Design review of the part built by this model. Coordinates are the model's own, in mm. Face numbers are marked on the shaded views. A direction names the side the tool comes from. Coordinates: 2 decimals unless noted, no trailing zeros. Loops run counter-clockwise (first coordinate to the right, second up) from the corner with the lowest first, then second, coordinate; pieces in that order, holes last. Notation, with made-up numbers: (6, 26) -> (35, 26) arc R23 ccw to (35, 53) -> close; hole circle Ø2 at (28, 63.25). An arc over 180 degrees is marked (long way). Answer in a Markdown table with one row per item.
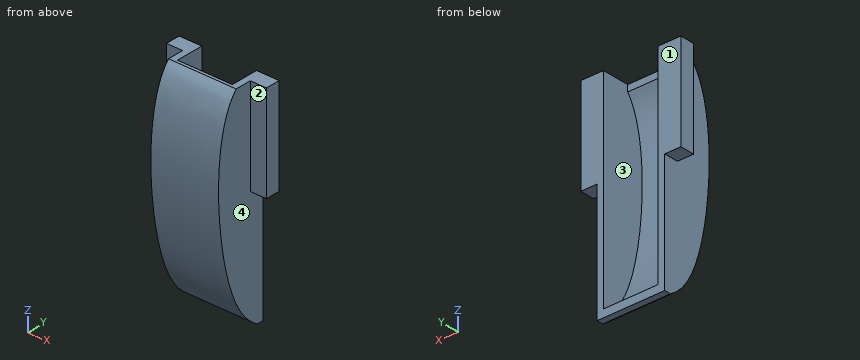
```python
from build123d import *

# Parameters (mm, degrees)
BASEPIEDEAPPOGGIO_START = -10.5
BASEPIEDEAPPOGGIO_DEPTH = 21
LATOSINISTRO_DEPTH      = 2
SCHIZZO3_W              = 5
SCHIZZO3_H              = 4.5
ALETTEAGGANCIO_DEPTH    = 30


# Read off the part's stored shape, not the designer's step: BasePiedeAppoggio
with BuildPart() as part:
    # BasePiedeAppoggio outline → BasePiedeAppoggio (new body)
    with BuildSketch(Plane(origin=(0, 0, 0), x_dir=(0, 0, -1), z_dir=(1, 0, 0)).offset(BASEPIEDEAPPOGGIO_START)):
        with BuildLine():
            Line((-67, -6.58541733), (-67, -7.5))
            add(Edge.make_bspline(
                [(-67, -7.5), (-60, -14), (-44, -17), (-14, -13), (-5, -8), (0, 0)],
                knots=[0, 0, 0, 0, 0, 0, 1, 1, 1, 1, 1, 1], degree=5))
            Line((0, 0), (0, 2))
            Line((0, 2), (-2.409917527, 2))
            Line((-2.409917527, 2), (-2.409917527, 0))
            add(Edge.make_bspline(
                [(-2.409917527, 0), (-2.667324323, -0.353402954), (-3.476108464, -1.377540434), (-5.718312008, -3.574118885), (-10.497685703, -6.435761001), (-19.037438877, -9.233820798), (-29.572047533, -11.136431528), (-38.966676556, -11.799385995), (-46.135832891, -11.693755764), (-51.166703498, -11.28631183), (-55.693282116, -10.549034431), (-58.932001396, -9.671882802), (-61.157085706, -8.829738395), (-62.633910182, -8.137838289), (-63.931461685, -7.382278902), (-64.645771008, -6.869387628), (-65, -6.58541733)],
                knots=[0.030225408, 0.030225408, 0.030225408, 0.030225408, 0.061229523, 0.122459046, 0.244918093, 0.367377139, 0.489836186, 0.612295232, 0.673524756, 0.734754279, 0.795983802, 0.857213325, 0.887828087, 0.918442849, 0.94905761, 0.979672372, 0.979672372, 0.979672372, 0.979672372], degree=3))
            Line((-65, -6.58541733), (-67, -6.58541733))
        make_face()
    extrude(amount=BASEPIEDEAPPOGGIO_DEPTH)

    # Schizzo2 → LatoSinistro (add)
    with BuildSketch(Plane.ZY.offset(10.5)):
        with BuildLine():
            Line((67, -7.5), (67, 2))
            Line((67, 2), (0, 2))
            Line((0, 2), (0, 0))
            add(Edge.make_bspline(
                [(67, -7.5), (60, -14), (44, -17), (14, -13), (5, -8), (0, 0)],
                knots=[0, 0, 0, 0, 0, 0, 1, 1, 1, 1, 1, 1], degree=5))
        make_face()
    latosinistro = extrude(amount=-LATOSINISTRO_DEPTH)

    # LatoDestro: LatoSinistro across plane
    add(latosinistro.mirror(Plane(origin=(0, 0, 0), x_dir=(0, 0, 1), z_dir=(1, 0, 0))))

    # Schizzo3 → AletteAggancio (add)
    with BuildSketch(Plane.XY.offset(67)):
        with Locations((-13, -0.25)):
            Rectangle(SCHIZZO3_W, SCHIZZO3_H)
        with Locations((13, -0.25)):
            Rectangle(SCHIZZO3_W, SCHIZZO3_H)
    extrude(amount=-ALETTEAGGANCIO_DEPTH)


solid = part.part
```
(1) Tool access review of the marked faces 1 and 2: name each direction out of +Z, -Z, +X, -X, +Y, -Y from which nothing blocks a thin tool from reaching the whole face with its end or side.
Evaluation:
| item | result |
|---|---|
| face 1 | +Z, -Z, +X, -X, +Y |
| face 2 | +Z, -Z, +X, -Y |
(2) To check wall thickness, follow probe 1 along X at (y, z) = (-7.75, 21); probe 2 along X at (y, z) = (-1.5, 62.5); probe 3 along Y at (x, z) = (13, 63). State the ranges of each line that lie inside material, in increasing order.
Evaluation:
| item | result |
|---|---|
| probe 1 | x = -10.5 to -8.5, 8.5 to 10.5 |
| probe 2 | x = -15.5 to -8.5, 8.5 to 15.5 |
| probe 3 | y = -2.5 to 2 |
(3) Draft analysis for pull direction Z (two halves, no side actions). For the marked faces 3 and 4, state which applies: pulls with the +Z half, pulls with the -Z half, needs draft (parallel to the pull), parting line crosses it, or undercut.
Evaluation:
| item | result |
|---|---|
| face 3 | undercut |
| face 4 | needs draft |
(4) Take a section at A-A on x = 12.5. Give the boundary of the cut face in (y, z).
Evaluation:
| item | result |
|---|---|
| outline | (-2.5, 37) -> (2, 37) -> (2, 67) -> (-2.5, 67) -> close |
(5) For pin 1 (4 mm diameter, centred on y = -10, z = 57.5, fed in from -X); pin 2 (12 mm diameter, centred on x = 8.5, z = 26.5, fed in from -Y); pin 3 (1 mm diameter, centred on x = -0.5, y = 1.5, fed in from +Z), all flat-tipped, find the tip position at first contact; note any pin that passes through.
Evaluation:
| item | result |
|---|---|
| pin 1 | stops at x = -10.5 |
| pin 2 | stops at y = -13.27 |
| pin 3 | stops at z = 2.41 |
